from build123d import *

# Parameters (mm, degrees)
F1_DEPTH = 15.875
F2_R     = 1.1303
F3_DEPTH = 15.876


with BuildPart() as f1:
    # F0 (on Top) → F1 (new body)
    with BuildSketch(Plane.XY):
        Polygon((3.4925, 1.446641), (1.446641, 3.4925), (-1.446641, 3.4925), (-3.4925, 1.446641), (-3.4925, -1.446641), (-1.446641, -3.4925), (1.446641, -3.4925), (3.4925, -1.446641), align=None)
    extrude(amount=F1_DEPTH)

    # F2 (on Top) → F3 (cut, through all)
    with BuildSketch(Plane.XY):
        Circle(F2_R)
    extrude(amount=F3_DEPTH, mode=Mode.SUBTRACT)


solid = f1.part
Check sheet for the modelled part. Datum: model origin and axes. Units: mm. Round coordinates to 2 decimals unless told otherwise and drop trailing zeros. Order: outer loops, then holes, each group sorted by start corner. A loop starts at its lowest first (then second) coordinate and runs counter-clockwise, first axis right, second up.
Q1. Cross-section at B-B, the plane y = 0. Enter the section's corners in (x, z) (1 decimal), plus the area to 3 significant figures.
Filled sheet:
outline: (-3.5, 0) - (-1.1, 0) - (-1.1, 15.9) - (-3.5, 15.9) - close; (1.1, 0) - (3.5, 0) - (3.5, 15.9) - (1.1, 15.9) - close
area: 75.0 mm2
Q2. Depth check by flat-ended pin: P1, Ø1.5, axis at y = 2.5, z = 11.5, coming from the +X side. Enter the tip coordinate at first touch or a pass-through.
Filled sheet:
P1: stops at x = 3.19
Q3. Draft check along Y on faces 1 (the face through (-1, 1, 0)), 2 (the face through (-2.48, -2.46, 7.83)), 3 (the face through (-0.245, -1.103, 7.826)). Enter one of: pulls with the +Y half, pulls with the -Y half, needs draft (parallel to the pull), parting line crosses it, or undercut.
Filled sheet:
face 1: needs draft
face 2: pulls with the -Y half
face 3: undercut
Q4. Cross-section at D-D, the plane x = 1.75. Enter the section's corners in (y, z) (3 decimals), plus the area to 3 significant figures.
Filled sheet:
outline: (-3.189, 0) - (3.189, 0) - (3.189, 15.875) - (-3.189, 15.875) - close
area: 101 mm2
Q5. Cross-section at A-A, the plane z = 9.5. Enter the section's corners in (x, y).
Filled sheet:
outline: (-3.49, -1.45) - (-1.45, -3.49) - (1.45, -3.49) - (3.49, -1.45) - (3.49, 1.45) - (1.45, 3.49) - (-1.45, 3.49) - (-3.49, 1.45) - close; hole circle Ø2.26 at (0, 0)
Q6. Scan lines: L1, parallel to Y at x = 0, z = 11.25; L2, parallel to Y at x = -1, z = 5.25. Record each from-to range of solid material in increasing order.
Filled sheet:
L1: y = -3.49 to -1.13, 1.13 to 3.49
L2: y = -3.49 to -0.53, 0.53 to 3.49
